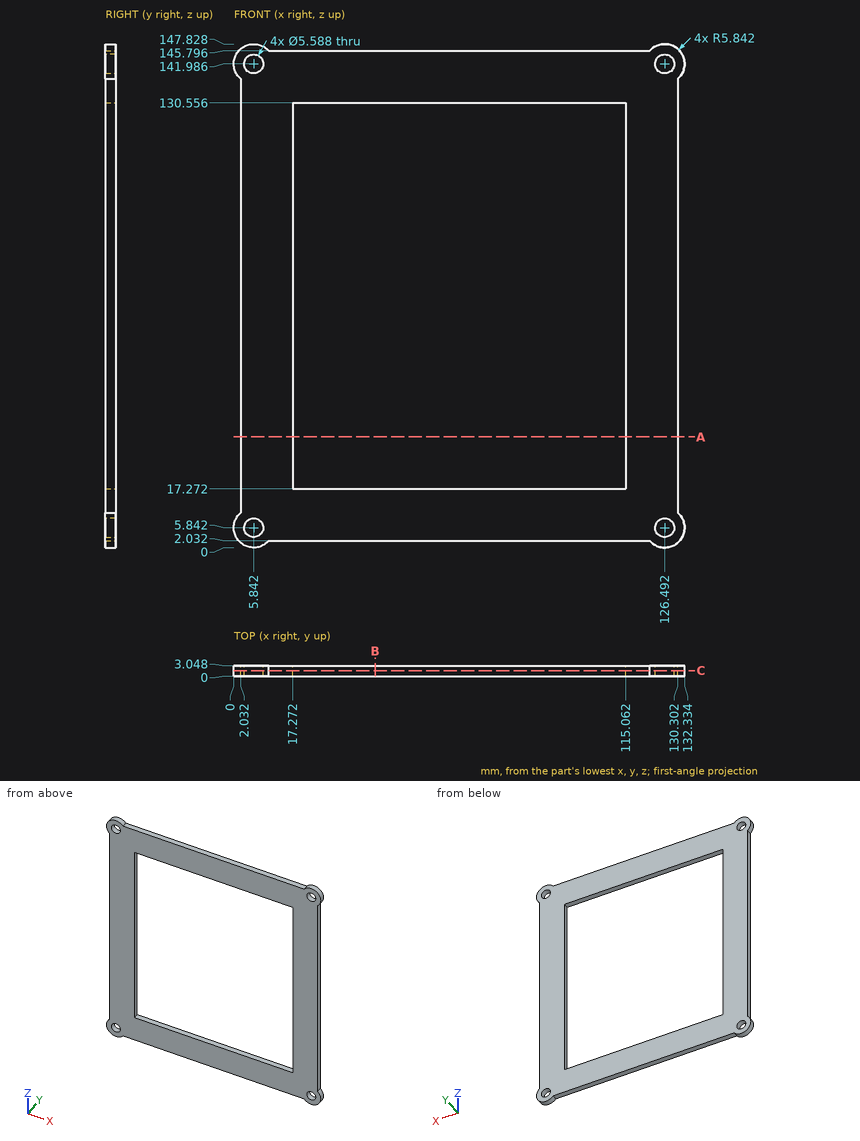
Can you work these out from the drawing? Everything is in mm from the part's minimum corner. Coordinates: 2 decimals unless noted, no trailing zeros. Write each loop counter-clockwise with the first axis right and the second up, starting at its lowest first coordinate (ties: lowest second). Pieces come first, ordered by that corner, then holes. Notation, with made-up numbers: (-1.5, 28) -> (46.5, 28) arc R32 ccw to (46.5, 67) -> close; hole circle Ø11 at (47, 58). An arc over 180 degrees is marked (long way). Write each question's results on one line, items separated by ' | '. Start each with the question number.
Q1. Imagine slicing it at B-B (x = 41.5). Write out the boundary of the cut face in (y, z), then the cut area to 3 significant figures.
Q2. Imagine slicing it at C-C (y = 1.6). Write out the boundary of the cut face in (x, z).
Q3. Imagine slicing it at A-A (z = 32.5). Write out the boundary of the cut face in (x, y), then the cut area to 3 significant figures.
Q4. If I drill on probe 1 along Z at (x, y) = (74, 1.95); probe 2 along X at (y, z) = (1.2, 46); probe 3 along X at (y, z) = (0.25, 8), over which ranges is the centre line in solid material (lowest first)?
Q5. I'm going to push flat-ended pins straight in: pin 1 (0.9 mm diameter, centred on y = 1.5, z = 76.5, fed in from -X); pin 2 (0.9 mm diameter, centred on x = 71.5, y = 2, fed in from -Z). Where does each tip first touch, or does it pass through?
Taken from the geometry:
1) outline: (0, 2.03) -> (3.05, 2.03) -> (3.05, 17.27) -> (0, 17.27) -> close; (0, 130.56) -> (3.05, 130.56) -> (3.05, 145.8) -> (0, 145.8) -> close | area: 92.9 mm^2
2) outline: (2.03, 10.27) arc R5.84 ccw (long way) to (10.27, 2.03) -> (122.06, 2.03) arc R5.84 ccw (long way) to (130.3, 10.27) -> (130.3, 137.56) arc R5.84 ccw (long way) to (122.06, 145.8) -> (10.27, 145.8) arc R5.84 ccw (long way) to (2.03, 137.56) -> close; hole circle Ø5.59 at (5.84, 5.84); hole circle Ø5.59 at (5.84, 141.99); hole (17.27, 17.27) -> (115.06, 17.27) -> (115.06, 130.56) -> (17.27, 130.56) -> close; hole circle Ø5.59 at (126.49, 5.84); hole circle Ø5.59 at (126.49, 141.99)
3) outline: (2.03, 0) -> (17.27, 0) -> (17.27, 3.05) -> (2.03, 3.05) -> close; (115.06, 0) -> (130.3, 0) -> (130.3, 3.05) -> (115.06, 3.05) -> close | area: 92.9 mm^2
4) probe 1: z = 2.03 to 17.27, 130.56 to 145.8 | probe 2: x = 2.03 to 17.27, 115.06 to 130.3 | probe 3: x = 0.41 to 4.07, 7.62 to 124.72, 128.27 to 131.92
5) pin 1: stops at x = 2.03 | pin 2: stops at z = 2.03
